from build123d import *

# Parameters (mm, degrees)
ESQUISSE1_R             = 2
BOSS_EXTRU_1_DEPTH      = 5
CHANFREIN1_SIZE         = 2
ENL_V_MAT_EXTRU_1_DEPTH = 2.5


with BuildPart() as part:
    # Esquisse1 → Boss.-Extru.1 (new body)
    with BuildSketch(Plane(origin=(0, 0, 0), x_dir=(1, 0, 0), z_dir=(0, 1, 0))):
        with BuildLine():
            Line((60, 14), (60, -14))
            ThreePointArc((60, -14), (58.242640687, -18.242640687), (54, -20))
            Line((54, -20), (41, -20))
            ThreePointArc((41, -20), (36.757359313, -21.757359313), (35, -26))
            Line((35, -26), (35, -44))
            ThreePointArc((35, -44), (33.242640687, -48.242640687), (29, -50))
            Line((29, -50), (-29, -50))
            ThreePointArc((-29, -50), (-33.242640687, -48.242640687), (-35, -44))
            Line((-35, -44), (-35, -26))
            ThreePointArc((-35, -26), (-36.757359313, -21.757359313), (-41, -20))
            Line((-41, -20), (-54, -20))
            ThreePointArc((-54, -20), (-58.242640687, -18.242640687), (-60, -14))
            Line((-60, -14), (-60, 14))
            ThreePointArc((-60, 14), (-58.242640687, 18.242640687), (-54, 20))
            Line((-54, 20), (-41, 20))
            ThreePointArc((-41, 20), (-36.757359313, 21.757359313), (-35, 26))
            Line((-35, 26), (-35, 44))
            ThreePointArc((-35, 44), (-33.242640687, 48.242640687), (-29, 50))
            Line((-29, 50), (29, 50))
            ThreePointArc((29, 50), (33.242640687, 48.242640687), (35, 44))
            Line((35, 44), (35, 26))
            ThreePointArc((35, 26), (36.757359313, 21.757359313), (41, 20))
            Line((41, 20), (54, 20))
            ThreePointArc((54, 20), (58.242640687, 18.242640687), (60, 14))
        make_face()
        with Locations(Location((20, -10, 0), (0, 0, 90))):
            Circle(ESQUISSE1_R, mode=Mode.SUBTRACT)
        with Locations(Location((-20, -10, 0), (0, 0, 270))):
            Circle(ESQUISSE1_R, mode=Mode.SUBTRACT)
        with Locations(Location((-54, -14, 0), (0, 0, 270))):
            Circle(ESQUISSE1_R, mode=Mode.SUBTRACT)
        with Locations(Location((20, 10, 0), (0, 0, 270))):
            Circle(ESQUISSE1_R, mode=Mode.SUBTRACT)
        with Locations(Location((-20, 10, 0), (0, 0, 90))):
            Circle(ESQUISSE1_R, mode=Mode.SUBTRACT)
        with Locations(Location((-41.5, -14, 0), (0, 0, 270))):
            Circle(ESQUISSE1_R, mode=Mode.SUBTRACT)
        with Locations(Location((-29, -29, 0), (0, 0, 270))):
            Circle(ESQUISSE1_R, mode=Mode.SUBTRACT)
        with Locations(Location((54, -14, 0), (0, 0, 90))):
            Circle(ESQUISSE1_R, mode=Mode.SUBTRACT)
        with Locations(Location((41.5, -14, 0), (0, 0, 90))):
            Circle(ESQUISSE1_R, mode=Mode.SUBTRACT)
        with Locations(Location((29, -29, 0), (0, 0, 90))):
            Circle(ESQUISSE1_R, mode=Mode.SUBTRACT)
        with BuildLine():
            Line((35, -2), (32, -2))
            ThreePointArc((32, -2), (30, 0), (32, 2))
            Line((32, 2), (35, 2))
            ThreePointArc((35, 2), (37, 0), (35, -2))
        make_face(mode=Mode.SUBTRACT)
        with BuildLine():
            Line((13, -14), (13, 14))
            ThreePointArc((13, 14), (11.242640687, 18.242640687), (7, 20))
            Line((7, 20), (-7, 20))
            ThreePointArc((-7, 20), (-11.242640687, 18.242640687), (-13, 14))
            Line((-13, 14), (-13, -14))
            ThreePointArc((-13, -14), (-11.242640687, -18.242640687), (-7, -20))
            Line((-7, -20), (7, -20))
            ThreePointArc((7, -20), (11.242640687, -18.242640687), (13, -14))
        make_face(mode=Mode.SUBTRACT)
        with BuildLine():
            Line((-18.1, -34.25451696), (-15.099999825, -34.25451696))
            ThreePointArc((-15.099999825, -34.25451696), (-13.1, -36.25451696), (-15.099999825, -38.25451696))
            Line((-15.099999825, -38.25451696), (-18.1, -38.25451696))
            ThreePointArc((-18.1, -38.25451696), (-20.1, -36.25451696), (-18.1, -34.25451696))
        make_face(mode=Mode.SUBTRACT)
        with BuildLine():
            Line((-35, -2), (-32, -2))
            ThreePointArc((-32, -2), (-30, 0), (-32, 2))
            Line((-32, 2), (-35, 2))
            ThreePointArc((-35, 2), (-37, 0), (-35, -2))
        make_face(mode=Mode.SUBTRACT)
        with BuildLine():
            Line((18.1, -34.25451696), (15.099999825, -34.25451696))
            ThreePointArc((15.099999825, -34.25451696), (13.1, -36.25451696), (15.099999825, -38.25451696))
            Line((15.099999825, -38.25451696), (18.1, -38.25451696))
            ThreePointArc((18.1, -38.25451696), (20.1, -36.25451696), (18.1, -34.25451696))
        make_face(mode=Mode.SUBTRACT)
        with BuildLine():
            Line((-18.1, 38.25451696), (-15.099999825, 38.25451696))
            ThreePointArc((-15.099999825, 38.25451696), (-13.1, 36.25451696), (-15.099999825, 34.25451696))
            Line((-15.099999825, 34.25451696), (-18.1, 34.25451696))
            ThreePointArc((-18.1, 34.25451696), (-20.1, 36.25451696), (-18.1, 38.25451696))
        make_face(mode=Mode.SUBTRACT)
        with BuildLine():
            Line((18.1, 38.25451696), (15.099999825, 38.25451696))
            ThreePointArc((15.099999825, 38.25451696), (13.1, 36.25451696), (15.099999825, 34.25451696))
            Line((15.099999825, 34.25451696), (18.1, 34.25451696))
            ThreePointArc((18.1, 34.25451696), (20.1, 36.25451696), (18.1, 38.25451696))
        make_face(mode=Mode.SUBTRACT)
    extrude(amount=BOSS_EXTRU_1_DEPTH)

    # Chanfrein1
    chanfrein1_edges = [part.edges().sort_by_distance(p)[0] for p in [
        (20, 5, 12),
        (-20, 5, 8),
        (20, 5, -12),
        (-20, 5, -8),
        (-54, 5, 12),
        (-41.5, 5, 12),
        (-29, 5, 27),
        (54, 5, 16),
        (41.5, 5, 16),
        (29, 5, 31),
    ]]
    chamfer(chanfrein1_edges, length=CHANFREIN1_SIZE)

    # Esquisse2 → Enlèv. mat.-Extru.1 (cut)
    with BuildSketch(Plane.XZ):
        with BuildLine():
            Line((-18.1, -32.25451696), (-15.1, -32.25451696))
            ThreePointArc((-15.1, -32.25451696), (-11.1, -36.25451696), (-15.1, -40.25451696))
            Line((-15.1, -40.25451696), (-18.1, -40.25451696))
            ThreePointArc((-18.1, -40.25451696), (-22.1, -36.25451696), (-18.1, -32.25451696))
        make_face()
        with BuildLine():
            Line((-18.1, 40.25451696), (-15.1, 40.25451696))
            ThreePointArc((-15.1, 40.25451696), (-11.1, 36.25451696), (-15.1, 32.25451696))
            Line((-15.1, 32.25451696), (-18.1, 32.25451696))
            ThreePointArc((-18.1, 32.25451696), (-22.1, 36.25451696), (-18.1, 40.25451696))
        make_face()
        with BuildLine():
            Line((18.1, 32.25451696), (15.1, 32.25451696))
            ThreePointArc((15.1, 32.25451696), (11.1, 36.25451696), (15.1, 40.25451696))
            Line((15.1, 40.25451696), (18.1, 40.25451696))
            ThreePointArc((18.1, 40.25451696), (22.1, 36.25451696), (18.1, 32.25451696))
        make_face()
        with BuildLine():
            Line((18.1, -40.25451696), (15.1, -40.25451696))
            ThreePointArc((15.1, -40.25451696), (11.1, -36.25451696), (15.1, -32.25451696))
            Line((15.1, -32.25451696), (18.1, -32.25451696))
            ThreePointArc((18.1, -32.25451696), (22.1, -36.25451696), (18.1, -40.25451696))
        make_face()
    extrude(amount=-ENL_V_MAT_EXTRU_1_DEPTH, mode=Mode.SUBTRACT)


solid = part.part
The listing builds one solid part. Answer for the finished solid, in the listing's coordinates (mm). A direction names the side the tool comes from. Round coordinates to 2 decimals unless told otherwise and drop trailing zeros. Write each loop counter-clockwise with the first axis right and the second up, starting at its lowest first coordinate (ties: lowest second). Pieces come first, ordered by that corner, then holes. Notation, with made-up numbers: M 76.5,88.5 L 80.5,88.5 A18 cw 80.5,103.5 Z; hole C -11,1.5 d8. An arc over 180 degrees is marked long. Write each question's results on one line, items separated by ' | '. Start each with the question number.
Item 1: Straight lines are drawn through the part: L1, parallel to X at y = 1.2, z = 29; L2, parallel to X at y = 1.3, z = 14; L3, parallel to Z at x = 4, y = 2.85. For each, find the intervals that lie inside material, in ascending order. Write a range as [from, to].
Item 2: A cutting plane is placed at C-C on z = -0.5. Write down the section's boundary in (x, y).
Item 3: Flat-ended cylindrical pins translate along their axes: pin 1 Ø1 at (y, z) = (4, -38.5) entering from +X; pin 2 Ø6.5 at (x, z) = (41.5, 14) entering from +Y; pin 3 Ø1 at (y, z) = (2.5, -15.5) entering from +X. Find the tip coordinate at first contact, or state that the pin passes through.
Item 4: For faces 4 (the face through (33, 2, -2)), 5 (the face through (-22.1, 1.2, -36.3)), 6 (the face through (58.289, 2.465, 18.196)), determine the directions among +Z, -Z, +X, -X, +Y, -Y from which every point of the face is accessible in a straight line to the end or side of a thin tool.
Item 5: A cutting plane is placed at B-B on y = 4.1. State how many separate pieces and enclosed holes the cut face has, and give its area (3 significant figures).
Item 6: A cutting plane is placed at A-A on z = 29. Write down the section's boundary in (x, y).
Item 7: For a pull along Z with two mould halves and no side action, classify faces 1 (the face through (36.711, 2.465, -21.804)), 2 (the face through (-18, 1, 10)), 3 (the face through (33.289, 2.465, 48.196)) as pulls with the +Z half, pulls with the -Z half, needs draft (parallel to the pull), parting line crosses it, or undercut.
Item 8: A cutting plane is placed at D-D on z = -30. Write down the section's boundary in (x, y).
Check sheet entries:
1) L1: [-35, -31], [-27, 27], [31, 35] | L2: [-60, -56], [-52, -43.5], [-39.5, -13], [13, 39.5], [43.5, 52], [56, 60] | L3: [-50, -20], [20, 50]
2) outline: M -60,0 L -36.94,0 L -36.94,5 L -60,5 Z; M -30.06,0 L -13,0 L -13,5 L -30.06,5 Z; M 13,0 L 30.06,0 L 30.06,5 L 13,5 Z; M 36.94,0 L 60,0 L 60,5 L 36.94,5 Z
3) pin 1: x = 35 | pin 2: y = 4.25 | pin 3: x = 59.92
4) face 4: +Y, -Y | face 5: -Y | face 6: +Z, +X, +Y, -Y
5) separate pieces: 1 | enclosed holes: 17 | area: 7,510 mm²
6) outline: M -35,0 L -31,0 L -31,3 L -33,5 L -35,5 Z; M -27,0 L 27,0 L 27,3 L 25,5 L -25,5 L -27,3 Z; M 31,0 L 35,0 L 35,5 L 33,5 L 31,3 Z
7) face 1: pulls with the -Z half | face 2: undercut | face 3: pulls with the +Z half
8) outline: M -35,0 L 35,0 L 35,5 L -35,5 Z
